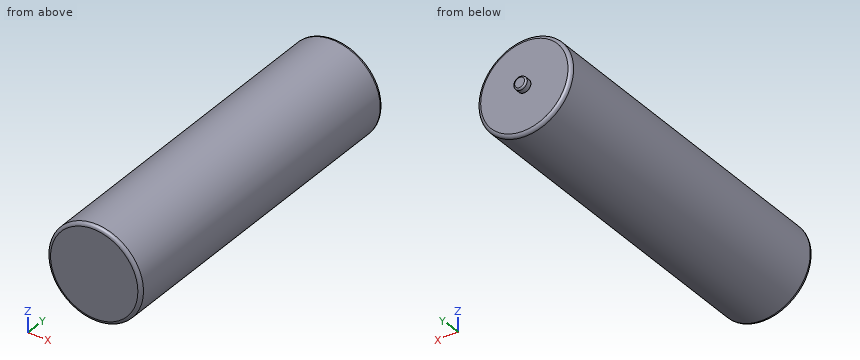
```python
from build123d import *

# Parameters (mm, degrees)
SKETCH1_R           = 7.175
BOSS_EXTRUDE1_DEPTH = 51
FILLET1_R           = 0.5
SKETCH2_R           = 1
BOSS_EXTRUDE2_DEPTH = 1
FILLET2_R           = 0.25


with BuildPart() as part:
    # Sketch1 → Boss-Extrude1 (new body)
    with BuildSketch(Plane(origin=(0, 0, 0), x_dir=(1, 0, 0), z_dir=(0, 1, 0))):
        Circle(SKETCH1_R)
    extrude(amount=BOSS_EXTRUDE1_DEPTH)

    # Fillet1
    fillet1_edges = [part.edges().sort_by_distance(p)[0] for p in [
        (-7.175, 0, 0),
        (-7.175, 51, 0),
    ]]
    fillet(fillet1_edges, radius=FILLET1_R)

    # Sketch2 → Boss-Extrude2 (add)
    with BuildSketch(Plane(origin=(0, 51, 0), x_dir=(1, 0, 0), z_dir=(0, 1, 0))):
        Circle(SKETCH2_R)
    extrude(amount=BOSS_EXTRUDE2_DEPTH)

    # Fillet2
    fillet2_edges = [part.edges().sort_by_distance(p)[0] for p in [
        (-1, 52, 0),
    ]]
    fillet(fillet2_edges, radius=FILLET2_R)


solid = part.part
```
Could you check a few things on this model? Use its own coordinates, in mm. Round coordinates to 2 decimals unless told otherwise and drop trailing zeros. Loops run counter-clockwise (first coordinate to the right, second up) from the corner with the lowest first, then second, coordinate; pieces in that order, holes last. Notation, with made-up numbers: (75, 72.25) -> (99, 72.25) arc R9 cw to (99, 77.25) -> close; hole circle Ø8 at (-27.75, -17). An arc over 180 degrees is marked (long way). One line per question, with ' | ' between items.
(1) If we section it at A-A on z = 0: List the corners of the cut face in (x, y) for me (3 decimals).
Model answer:
outline: (-7.175, 0.5) arc R0.5 ccw to (-6.675, 0) -> (6.675, 0) arc R0.5 ccw to (7.175, 0.5) -> (7.175, 50.5) arc R0.5 ccw to (6.675, 51) -> (1, 51) -> (1, 51.75) arc R0.25 ccw to (0.75, 52) -> (-0.75, 52) arc R0.25 ccw to (-1, 51.75) -> (-1, 51) -> (-6.675, 51) arc R0.5 ccw to (-7.175, 50.5) -> close
(2) If I drill on probe 1 along Y at (x, z) = (-5.5, 3); probe 2 along X at (y, z) = (29.5, -0.25); probe 3 along X at (y, z) = (11.5, -3.5), over which ranges is the centre line in solid material (lowest first)?
Model answer:
probe 1: y = 0 to 51 | probe 2: x = -7.17 to 7.17 | probe 3: x = -6.26 to 6.26
(3) If we section it at C-C on y = 44.5: List the corners of the cut face in (x, z) for me (3 decimals), and give its area (3 significant figures).
Model answer:
outline: circle Ø14.35 at (0, 0) | area: 162 mm^2
(4) For pin 1 Ø5 at (x, z) = (-4, 3.5) entering from +Y, with a flat end and sliding along its axis, tell me the tip position at first contact or that it passes through.
Model answer:
pin 1: stops at y = 51
(5) If we section it at B-B on x = 0: List the corners of the cut face in (y, z) for me (3 decimals), and give its area (3 significant figures).
Model answer:
outline: (0, -6.675) arc R0.5 ccw to (0.5, -7.175) -> (50.5, -7.175) arc R0.5 ccw to (51, -6.675) -> (51, -1) -> (51.75, -1) arc R0.25 ccw to (52, -0.75) -> (52, 0.75) arc R0.25 ccw to (51.75, 1) -> (51, 1) -> (51, 6.675) arc R0.5 ccw to (50.5, 7.175) -> (0.5, 7.175) arc R0.5 ccw to (0, 6.675) -> close | area: 734 mm^2
